Geometry check sheet. Reference: the model listing, model coordinates, mm. Round coordinates to 2 decimals unless told otherwise and drop trailing zeros. Order: outer loops, then holes, each group sorted by start corner. A loop starts at its lowest first (then second) coordinate and runs counter-clockwise, first axis right, second up. Notation, with made-up numbers: (89.25, 8.5) -> (119.25, 8.5) arc R13 ccw to (119.25, 14.5) -> close; hole circle Ø9 at (48.5, -22). An arc over 180 degrees is marked (long way). Use a Markdown table: item, result. Add a question column.
Item 1: Sectioned sample at B-B, the plane x = -8. Record the cut outline in (y, z), and give its area (3 significant figures).
Item 2: Gauge pin test, flat ends, axial feed: pin 1 Ø3 at (x, z) = (-20.58, 65.28) entering from -Y; pin 2 Ø6 at (x, z) = (46.25, 50.47) entering from -Y. Record the tip position at first contact, or that the pin passes through.
Item 3: Sectioned sample at D-D, the plane x = -59. Record the cut outline in (y, z).
Item 4: Sectioned sample at C-C, the plane z = -18.5. Record the cut outline in (x, y), and give its area (3 significant figures).
Item 5: Material ranges on probe 1 along Z at (x, y) = (0, -76.6); probe 2 along Z at (x, y) = (-38.5, -75.85); probe 3 along Z at (x, y) = (-42, -77.3), recorded low to high. Write a range as [from, to].
Item 6: Sectioned sample at A-A, the plane z = -38. Record the cut outline in (x, y).
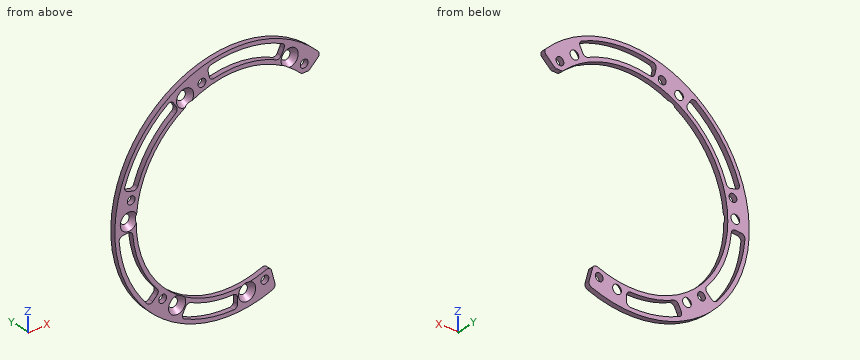
from build123d import *

# Parameters (mm, degrees)
BOSS_EXTRUDE1_DEPTH                          = 3.175
F_10_CLEARANCE_HOLE1_D                       = 5.1054
F_10_CLEARANCE_HOLE1_DEPTH                   = 3.175
CSK_FOR_10_FLAT_HEAD_MACHINE_SCREW1_AT_COUNT = 2
CSK_FOR_10_FLAT_HEAD_MACHINE_SCREW1_AT_PITCH = 46.824609742
CSK_FOR_10_FLAT_HEAD_MACHINE_SCREW1_2_COUNT  = 2
CSK_FOR_10_FLAT_HEAD_MACHINE_SCREW1_2_PITCH  = 104.87608053
CSK_FOR_10_FLAT_HEAD_MACHINE_SCREW1_3_COUNT  = 2
CSK_FOR_10_FLAT_HEAD_MACHINE_SCREW1_3_PITCH  = 134.826090234
CSK_FOR_10_FLAT_HEAD_MACHINE_SCREW1_4_COUNT  = 2
CSK_FOR_10_FLAT_HEAD_MACHINE_SCREW1_4_PITCH  = 128.649557941
FILLET1_R                                    = 2.54
CUT_EXTRUDE1_REACH                           = 5.175


with BuildPart() as part:
    # Sketch6 → Boss-Extrude1 (new body)
    with BuildSketch(Plane(origin=(0, -75.25766, 0), x_dir=(1, 0, 0), z_dir=(0, 1, 0))):
        with BuildLine():
            ThreePointArc((27.776705308, 72.346331375), (-75.433008797, -17.75945396), (57.135602127, -52.355133375))
            Line((57.135602127, -52.355133375), (49.374216067, -45.243133375))
            Line((49.374216067, -45.243133375), (44.556805119, -45.243133375))
            ThreePointArc((44.556805119, -45.243133375), (-62.309050026, -12.240599855), (24.13, 58.736641886))
            Line((24.13, 58.736641886), (27.776705308, 72.346331375))
        make_face()
    extrude(amount=-BOSS_EXTRUDE1_DEPTH)

    # #10 Clearance Hole1
    with Locations(Plane(origin=(0, -75.25766, 0), x_dir=(1, 0, 0), z_dir=(0, 1, 0))):
        with Locations((-46.246176482, 50.468845537), (20.584214093, 65.28478643), (-66.830390575, -14.815940893), (-20.584214093, -65.28478643), (46.246176482, -50.468845537)):
            Hole(F_10_CLEARANCE_HOLE1_D / 2, depth=F_10_CLEARANCE_HOLE1_DEPTH)

    # Sketch10 → CSK for #10 Flat Head Machine Screw1 (revolve, cut)
    with BuildSketch(Plane(origin=(8.934909436, -78.43266, -67.867375096), x_dir=(0, 0, -1), z_dir=(1, 0, 0))):
        Polygon((0, 0), (0, 3.175), (2.5527, 3.175), (2.5527, 3.506322905), (5.6007, 0), align=None)
    csk_for_10_flat_head_machine_screw1 = revolve(axis=Axis((8.934909436, -84.78266, -67.867375096), (0, 1, 0)), mode=Mode.SUBTRACT)

    # CSK for #10 Flat Head Machine Screw1 at: CSK for #10 Flat Head Machine Screw1 ×2
    with Locations(*[Vector(-0.976296007, 0, 0.216439614) * (i * CSK_FOR_10_FLAT_HEAD_MACHINE_SCREW1_AT_PITCH) for i in range(1, CSK_FOR_10_FLAT_HEAD_MACHINE_SCREW1_AT_COUNT)]):
        add(csk_for_10_flat_head_machine_screw1, mode=Mode.SUBTRACT)

    # CSK for _10 Flat Head Machine Screw1 2: CSK for #10 Flat Head Machine Screw1 ×2
    with Locations(*[Vector(-0.737277337, 0, 0.675590208) * (i * CSK_FOR_10_FLAT_HEAD_MACHINE_SCREW1_2_PITCH) for i in range(1, CSK_FOR_10_FLAT_HEAD_MACHINE_SCREW1_2_COUNT)]):
        add(csk_for_10_flat_head_machine_screw1, mode=Mode.SUBTRACT)

    # CSK for _10 Flat Head Machine Screw1 3: CSK for #10 Flat Head Machine Screw1 ×2
    with Locations(*[Vector(-0.3007058, 0, 0.953716951) * (i * CSK_FOR_10_FLAT_HEAD_MACHINE_SCREW1_3_PITCH) for i in range(1, CSK_FOR_10_FLAT_HEAD_MACHINE_SCREW1_3_COUNT)]):
        add(csk_for_10_flat_head_machine_screw1, mode=Mode.SUBTRACT)

    # CSK for _10 Flat Head Machine Screw1 4: CSK for #10 Flat Head Machine Screw1 ×2
    with Locations(*[Vector(0.216439614, 0, 0.976296007) * (i * CSK_FOR_10_FLAT_HEAD_MACHINE_SCREW1_4_PITCH) for i in range(1, CSK_FOR_10_FLAT_HEAD_MACHINE_SCREW1_4_COUNT)]):
        add(csk_for_10_flat_head_machine_screw1, mode=Mode.SUBTRACT)

    # Fillet1
    fillet1_edges = [part.edges().sort_by_distance(p)[0] for p in [
        (24.13, -76.84516, -58.736641886),
        (27.776705308, -76.84516, -72.346331375),
        (57.135602127, -76.84516, 52.355133375),
        (49.374216067, -76.84516, 45.243133375),
        (44.556805119, -76.84516, 45.243133375),
    ]]
    fillet(fillet1_edges, radius=FILLET1_R)

    # Sketch14 → Cut-Extrude1 (cut, up to next)
    with BuildSketch(Plane(origin=(0, -75.25766, 0), x_dir=(1, 0, 0), z_dir=(0, 1, 0)), mode=Mode.PRIVATE) as cut_extrude1_sk1:
        with BuildLine():
            Line((-33.055101826, 64.380888472), (-31.302158707, 60.966709443))
            ThreePointArc((-31.302158707, 60.966709443), (-29.864658567, 59.723557233), (-27.966930931, 59.825850385))
            ThreePointArc((-27.966930931, 59.825850385), (-14.293672104, 64.47458831), (0.063150386, 66.039969806))
            ThreePointArc((0.063150386, 66.039969806), (1.826306674, 66.749275081), (2.603745418, 68.483467419))
            Line((2.603745418, 68.483467419), (2.749557011, 72.318590234))
            ThreePointArc((2.749557011, 72.318590234), (2.043811589, 74.174021303), (0.21880546, 74.955080637))
            ThreePointArc((0.21880546, 74.955080637), (-16.223317839, 73.178657732), (-31.87569098, 67.839902076))
            ThreePointArc((-31.87569098, 67.839902076), (-33.199618308, 66.360741002), (-33.055101826, 64.380888472))
        make_face()
    cut_extrude1_tool1 = extrude(cut_extrude1_sk1.sketch, amount=-CUT_EXTRUDE1_REACH, mode=Mode.PRIVATE) & part.part
    add(cut_extrude1_tool1.solids().sort_by_distance((-15.117133, -75.25766, -68.188982))[0], mode=Mode.SUBTRACT)
    # Sketch14 → Cut-Extrude1 (cut, up to next)
    with BuildSketch(Plane(origin=(0, -75.25766, 0), x_dir=(1, 0, 0), z_dir=(0, 1, 0)), mode=Mode.PRIVATE) as cut_extrude1_sk2:
        with BuildLine():
            Line((-52.717941235, 49.581823576), (-49.92225926, 46.952452868))
            ThreePointArc((-49.92225926, 46.952452868), (-49.125502701, 45.22705058), (-49.749009498, 43.431758587))
            ThreePointArc((-49.749009498, 43.431758587), (-60.775101299, 25.839285248), (-65.794171702, 5.69285254))
            ThreePointArc((-65.794171702, 5.69285254), (-66.654447051, 3.998225622), (-68.449798516, 3.374890088))
            Line((-68.449798516, 3.374890088), (-72.283035848, 3.56388633))
            ThreePointArc((-72.283035848, 3.56388633), (-74.069896676, 4.42865765), (-74.688924078, 6.314792886))
            ThreePointArc((-74.688924078, 6.314792886), (-68.979739974, 29.327588756), (-56.36825574, 49.405786442))
            ThreePointArc((-56.36825574, 49.405786442), (-54.580464724, 50.268633089), (-52.717941235, 49.581823576))
        make_face()
    cut_extrude1_tool2 = extrude(cut_extrude1_sk2.sketch, amount=-CUT_EXTRUDE1_REACH, mode=Mode.PRIVATE) & part.part
    add(cut_extrude1_tool2.solids().sort_by_distance((-63.655179, -75.25766, -27.063786))[0], mode=Mode.SUBTRACT)
    # Sketch14 → Cut-Extrude1 (cut, up to next)
    with BuildSketch(Plane(origin=(0, -75.25766, 0), x_dir=(1, 0, 0), z_dir=(0, 1, 0)), mode=Mode.PRIVATE) as cut_extrude1_sk3:
        with BuildLine():
            Line((-69.2980894, -20.864164557), (-65.623146584, -19.7577183))
            ThreePointArc((-65.623146584, -19.7577183), (-63.730526092, -19.930408023), (-62.487511016, -21.368026745))
            ThreePointArc((-62.487511016, -21.368026745), (-52.76502809, -39.713139018), (-37.827240771, -54.132997845))
            ThreePointArc((-37.827240771, -54.132997845), (-36.789788484, -55.725331611), (-37.147639809, -57.591819355))
            Line((-37.147639809, -57.591819355), (-39.227934022, -60.817002142))
            ThreePointArc((-39.227934022, -60.817002142), (-40.870278368, -61.932083352), (-42.813233098, -61.52510919))
            ThreePointArc((-42.813233098, -61.52510919), (-59.888306882, -45.074412786), (-70.970794023, -24.113448217))
            ThreePointArc((-70.970794023, -24.113448217), (-70.824145631, -22.133752457), (-69.2980894, -20.864164557))
        make_face()
    cut_extrude1_tool3 = extrude(cut_extrude1_sk3.sketch, amount=-CUT_EXTRUDE1_REACH, mode=Mode.PRIVATE) & part.part
    add(cut_extrude1_tool3.solids().sort_by_distance((-55.265515, -75.25766, 41.595109))[0], mode=Mode.SUBTRACT)
    # Sketch14 → Cut-Extrude1 (cut, up to next)
    with BuildSketch(Plane(origin=(0, -75.25766, 0), x_dir=(1, 0, 0), z_dir=(0, 1, 0)), mode=Mode.PRIVATE) as cut_extrude1_sk4:
        with BuildLine():
            Line((-16.580148165, -70.445988133), (-15.700887324, -66.710171168))
            ThreePointArc((-15.700887324, -66.710171168), (-14.60502339, -65.157458603), (-12.738501518, -64.799785332))
            ThreePointArc((-12.738501518, -64.799785332), (8.010073209, -65.552424266), (27.966930931, -59.825850385))
            ThreePointArc((27.966930931, -59.825850385), (29.864658567, -59.723557233), (31.302158707, -60.966709443))
            Line((31.302158707, -60.966709443), (33.055101826, -64.380888472))
            ThreePointArc((33.055101826, -64.380888472), (33.199618308, -66.360741002), (31.87569098, -67.839902076))
            ThreePointArc((31.87569098, -67.839902076), (9.091433092, -74.402001542), (-14.602538283, -73.519234659))
            ThreePointArc((-14.602538283, -73.519234659), (-16.243680907, -72.402385546), (-16.580148165, -70.445988133))
        make_face()
    cut_extrude1_tool4 = extrude(cut_extrude1_sk4.sketch, amount=-CUT_EXTRUDE1_REACH, mode=Mode.PRIVATE) & part.part
    add(cut_extrude1_tool4.solids().sort_by_distance((8.389663, -75.25766, 68.658895))[0], mode=Mode.SUBTRACT)


solid = part.part
Found:
| question | item | result |
|---|---|---|
| 1 | outline | (-78.43, -77.08) -> (-75.26, -77.08) -> (-75.26, -74.53) -> (-78.43, -74.53) -> close; (-78.43, -65.55) -> (-75.26, -65.55) -> (-75.26, -62.99) -> (-78.43, -62.99) -> close; (-78.43, 62.99) -> (-75.26, 62.99) -> (-75.26, 65.55) -> (-78.43, 65.55) -> close; (-78.43, 74.53) -> (-75.26, 74.53) -> (-75.26, 77.08) -> (-78.43, 77.08) -> close |
| 1 | area | 32.5 mm2 |
| 2 | pin 1 | passes through |
| 2 | pin 2 | stops at y = -78.43 |
| 3 | outline | (-78.43, -50.24) -> (-75.26, -50.24) -> (-75.26, -46.23) -> (-78.43, -46.23) -> close; (-78.43, -29.67) -> (-75.26, -29.67) -> (-75.26, -23.48) -> (-78.43, -23.48) -> close; (-78.43, 23.48) -> (-75.26, 23.48) -> (-75.26, 29.67) -> (-78.43, 29.67) -> close; (-78.43, 46.23) -> (-75.26, 46.23) -> (-75.26, 50.24) -> (-78.43, 50.24) -> close |
| 4 | outline | (-75.25, -78.43) -> (-72.64, -78.43) -> (-72.64, -75.26) -> (-75.25, -75.26) -> close; (-63.4, -78.43) -> (-60.75, -78.43) -> (-60.75, -75.26) -> (-63.4, -75.26) -> close |
| 4 | area | 16.7 mm2 |
| 5 | probe 1 | z = [-77.5, -74.96], [-66.04, -63.5], [63.5, 66.04], [74.96, 77.5] |
| 5 | probe 2 | z = [-67.26, -60.61], [-54.85, -50.5], [50.5, 53.66], [59.69, 67.26] |
| 5 | probe 3 | z = [-65.13, -47.63], [47.63, 50.96], [61.9, 65.13] |
| 6 | outline | (-67.54, -78.43) -> (-64.61, -78.43) -> (-64.61, -75.26) -> (-67.54, -75.26) -> close; (-54.01, -78.43) -> (-50.87, -78.43) -> (-50.87, -75.26) -> (-54.01, -75.26) -> close |
